from build123d import *

# Parameters (mm, degrees)
SKETCH3_W               = 300
SKETCH3_H               = 7.83336639
CUT_EXTRUDE1_DEPTH      = 5
CUT_EXTRUDE1_DEPTH_BACK = 5
SKETCH4_R               = 1
CUT_EXTRUDE2_DEPTH      = 5
CUT_EXTRUDE2_DEPTH_BACK = 5


with BuildPart() as part:
    # Sketch2 → Revolve1 (revolve)
    with BuildSketch(Plane(origin=(0, 0, 0), x_dir=(0, 0, -1), z_dir=(1, 0, 0))):
        Polygon((125, 0), (125, 4), (122, 4), (122, 2), (-125, 2), (-125, 0), align=None)
    revolve(axis=Axis((0, 0, 125), (0, 0, -1)))

    # Sketch3 → Cut-Extrude1 (cut, two sides)
    with BuildSketch(Plane(origin=(0, 0, 0), x_dir=(0, 0, -1), z_dir=(1, 0, 0))) as cut_extrude1_sk:
        with Locations((-56, 0.150641661)):
            Rectangle(SKETCH3_W, SKETCH3_H)
    extrude(amount=CUT_EXTRUDE1_DEPTH, mode=Mode.SUBTRACT)
    extrude(cut_extrude1_sk.sketch, amount=-CUT_EXTRUDE1_DEPTH_BACK, mode=Mode.SUBTRACT)

    # Sketch4 → Cut-Extrude2 (cut, two sides)
    with BuildSketch(Plane(origin=(0, 0, 0), x_dir=(1, 0, 0), z_dir=(0, 1, 0))) as cut_extrude2_sk:
        with Locations((0, 95.7)):
            Circle(SKETCH4_R)
    extrude(amount=CUT_EXTRUDE2_DEPTH, mode=Mode.SUBTRACT)
    extrude(cut_extrude2_sk.sketch, amount=-CUT_EXTRUDE2_DEPTH_BACK, mode=Mode.SUBTRACT)


solid = part.part
Build history of the part. All positions in model axes, mm. A direction names the side the tool comes from. Give positions to 0.01 mm unless a question says otherwise; leave off trailing zeros. Order: outer loops, then holes, each group sorted by start corner. A loop starts at its lowest first (then second) coordinate and runs counter-clockwise, first axis right, second up. Notation, with made-up numbers: M 63,30.25 L 114,30.25 A17 ccw 114,38.25 Z; hole C 7.5,70.5 d2. An arc over 180 degrees is marked long. Use one line per item in the form item = value.
Q1. Slice it at A-A, the plane x = 0. Write the cut outline in (y, z), and give its area (3 significant figures).
Conclusion:
outline = M -4,-125 L 4,-125 L 4,-122 L 2,-122 L 2,-96.7 L -2,-96.7 L -2,-122 L -4,-122 Z; M -2,-94.7 L 2,-94.7 L 2,-94 L -2,-94 Z
area = 128 mm2
Q2. Slice it at D-D, the plane z = -117.5. Write the cut outline in (x, y).
Conclusion:
outline = C 0,0 d4
Q3. Which spindle directions (+Z, -Z, +X, -X, +Y, -Y) get a long thin tool onto all of the face, cutting with end or side? Do faces 1 (the cylindrical face through (0, -2, -108)), 2 (the cylindrical face through (-3.905, -0.867, -123.479)). Say none if no direction does.
Conclusion:
face_1 = +Z
face_2 = +Z, -Z
Q4. Wall check: probe 1 along Z at (x, y) = (0, -0.5); probe 2 along X at (y, z) = (-1.3, -95.7); probe 3 along X at (y, z) = (0.55, -95.7). Give the ranges that are in metal, low to high.
Conclusion:
probe_1 = -125 to -96.7, -94.7 to -94
probe_2 = -1.52 to -1, 1 to 1.52
probe_3 = -1.92 to -1, 1 to 1.92
Q5. Slice it at B-B, the plane y = -0.5. Write the cut outline in (x, z), and give its area (3 significant figures).
Conclusion:
outline = M -3.97,-125 L 3.97,-125 L 3.97,-122 L 1.94,-122 L 1.94,-94 L -1.94,-94 L -1.94,-122 L -3.97,-122 Z; hole C 0,-95.7 d2
area = 129 mm2
Q6. Pin check, flat tips, straight feed: P1, Ø3, axis at x = -2.5, z = -101.5, coming from the -Y side; P2, Ø4, axis at y = 2, z = -102, coming from the -X side; P3, Ø1.5, axis at y = 1.5, z = -114.5, coming from the -X side; P4, Ø3, axis at x = -2.5, y = 2, coming from the +Z side. Stop position of each tip, or through.
Conclusion:
P1 = -1.73
P2 = -2
P3 = -1.85
P4 = -94
Q7. Slice it at C-C, the plane z = -95.7. Write the cut outline in (x, y).
Conclusion:
outline = M -1,-1.73 L -1,1.73 A2 ccw Z; M 1,-1.73 A2 ccw 1,1.73 Z
